The listing builds one solid part. Answer for the finished solid, in the listing's coordinates (mm). Face numbers are marked on the shaded views. A direction names the side the tool comes from. Round coordinates to 2 decimals unless told otherwise and drop trailing zeros. Loops run counter-clockwise (first coordinate to the right, second up) from the corner with the lowest first, then second, coordinate; pieces in that order, holes last. Notation, with made-up numbers: (-6, 63) - (10, 63) arc R12 ccw to (10, 71) - close; hole circle Ø10 at (5.25, -35.75). An arc over 180 degrees is marked (long way). One line per item, written item: value.
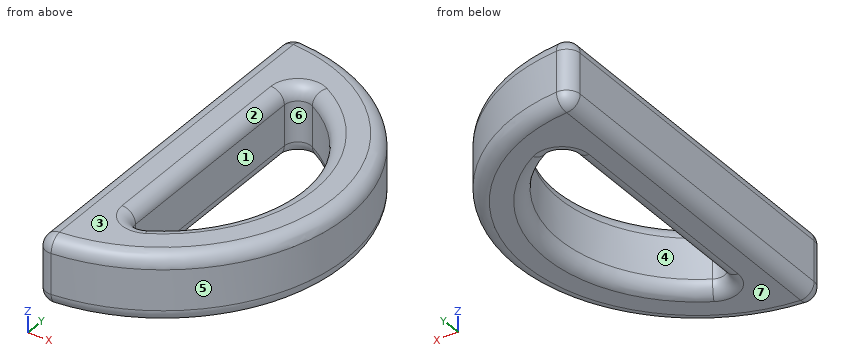
```python
from build123d import *

# Parameters (mm, degrees)
F1_DEPTH = 10
F2_R     = 2


with BuildPart() as f1:
    # F0 (on Top) → F1 (new body)
    with BuildSketch(Plane.XY):
        with BuildLine():
            Line((0, 7), (0, 0))
            ThreePointArc((0, 0), (27.5, 27.5), (0, 55))
            Line((0, 55), (0, 48))
            ThreePointArc((0, 48), (3.553808, 47.689612), (7, 46.767849))
            ThreePointArc((7, 46.767849), (20.5, 27.5), (7, 8.232151))
            ThreePointArc((7, 8.232151), (3.553808, 7.310388), (0, 7))
        make_face()
        with BuildLine():
            Line((0, 27.5), (0, 7))
            ThreePointArc((0, 7), (3.553808, 7.310388), (7, 8.232151))
            Line((7, 8.232151), (7, 27.5))
            Line((7, 27.5), (0, 27.5))
        make_face()
        with BuildLine():
            Line((0, 48), (0, 27.5))
            Line((0, 27.5), (7, 27.5))
            Line((7, 27.5), (7, 46.767849))
            ThreePointArc((7, 46.767849), (3.553808, 47.689612), (0, 48))
        make_face()
    extrude(amount=F1_DEPTH)

    # F2
    f2_edges = [f1.edges().sort_by_distance(p)[0] for p in [
        (0, 0, 5),
        (0, 55, 5),
        (27.5, 27.5, 0),
        (27.5, 27.5, 10),
        (20.5, 27.5, 10),
        (7, 27.5, 10),
        (0, 27.5, 10),
        (20.5, 27.5, 0),
        (0, 27.5, 0),
        (7, 27.5, 0),
        (7, 8.232151, 5),
        (7, 46.767849, 5),
    ]]
    fillet(f2_edges, radius=F2_R)


solid = f1.part
```
1) For a pull along Y with two mould halves and no side action, classify the marked faces 4, 5, 6 and 7 as released by +Y, released by -Y, zero draft, split by the parting line, or undercut.
Final values:
face 4: undercut
face 5: split by the parting line
face 6: undercut
face 7: zero draft
2) For the marked faces 1, 2 and 3, determine the directions among +Z, -Z, +X, -X, +Y, -Y from which every point of the face is accessible in a straight line to the end or side of a thin tool.
Final values:
face 1: +Z, -Z
face 2: +Z
face 3: +Z, +X, -X, +Y, -Y
3) Each of these flat-tipped pins is pushed along its axis until it touches: pin 1 Ø6 at (y, z) = (36, 3) entering from +X; pin 2 Ø2 at (y, z) = (21.5, 3) entering from +X; pin 3 Ø3 at (y, z) = (33, 5) entering from +X. Where does it stop, or does it pass through?
Final values:
pin 1: x = 26.94
pin 2: x = 27.04
pin 3: x = 27.21
4) A cutting plane is placed at A-A on z = 6.75. Give the vertices of the cut face in (x, y), and give its area (3 significant figures).
Final values:
outline: (0, 2.08) arc R2 ccw to (2.16, 0.08) arc R27.5 ccw to (2.16, 54.92) arc R2 ccw to (0, 52.92) - close; hole (7, 11.34) arc R2 ccw to (9.97, 9.59) arc R20.5 ccw to (9.97, 45.41) arc R2 ccw to (7, 43.66) - close
area: 812 mm2
5) A cutting plane is placed at B-B on z = 0.75. Give the vertices of the cut face in (x, y), and give its area (3 significant figures).
Final values:
outline: (0.44, 2.08) arc R1.56 ccw to (2.12, 0.52) arc R27.06 ccw to (2.12, 54.48) arc R1.56 ccw to (0.44, 52.92) - close; hole (6.56, 11.34) arc R2.44 ccw to (10.19, 9.21) arc R20.94 ccw to (10.19, 45.79) arc R2.44 ccw to (6.56, 43.66) - close
area: 714 mm2
6) Consider L1, parallel to X at y = 27, z = 5.25; L2, parallel to Y at x = 12.25, z = 5.5; L3, parallel to X at y = 23, z = 7. Determine where each line is inside the solid, lowest interval first.
Final values:
L1: 0 to 7, 20.49 to 27.5
L2: 2.88 to 11.06, 43.94 to 52.12
L3: 0 to 7, 20 to 27.13
